Geometry check sheet. Reference: the model listing, model coordinates, mm. A direction names the side the tool comes from. Round coordinates to 2 decimals unless told otherwise and drop trailing zeros. Order: outer loops, then holes, each group sorted by start corner. A loop starts at its lowest first (then second) coordinate and runs counter-clockwise, first axis right, second up.
(1) Sectioned sample at A-A (z = 2.5). Record the boundary of the cut face in (x, y).
(2) Material ranges on line 1 along X through (y, z) = (18.95, 6.25); line 2 along Y through (x, z) = (5, 1.75); line 3 along X through (y, z) = (14.5, 7.5), recorded low to high.
(3) Release check for a two-part mould opening along Y. For faces 4 (the face through (21, 22.3, 11)), 5 (the face through (22.4, 9, 6)), 6 (the face through (11, 11, 0)) record: +Y half, -Y half, draft (parallel to the pull), parting line (faces both ways), or undercut.
(4) Sectioned sample at C-C (y = 3). Record the boundary of the cut face in (x, z), plus the area to 3 significant figures.
(5) Sectioned sample at B-B (x = 19). Record the boundary of the cut face in (y, z).
(6) Go/stop test with flat-tipped pins: pin 1 (2 mm diameter, centred on x = -2.42, z = 6.25, fed in from -Y); pin 2 (4 mm diameter, centred on x = 24.5, z = 8, fed in from +Y); pin 3 (0.9 mm diameter, centred on x = 24.5, z = 7, fed in from -Y). Record where each tip stops, or that it passes through.
(7) Sectioned sample at D-D (x = 5.5). Record the boundary of the cut face in (y, z), plus the area to 3 significant figures.
(8) Set-up check for faces 1 (the face through (21, 22.3, 1)), 2 (the face through (12.35, 25.01, 1.29)), 3 (the face through (24, 5, 4.45)): record each of +Z, -Z, +X, -X, +Y, -Y from which the full face is reachable in a straight line by a thin tool's end or side.
from build123d import *

# Parameters (mm, degrees)
SKETCH_1_W          = 22.4
SKETCH_1_H          = 22.3
EXTRUDE_1_DEPTH     = 12.5
SKETCH_5_R          = 6.25
EXTRUDE_4_DEPTH     = 5.5
SKETCH_6_R          = 2.35
EXTRUDE_5_DEPTH     = 3.7
SKETCH_10_W         = 12.5
SKETCH_10_H         = 2.5
EXTRUDE_8_DEPTH     = 4.7
SKETCH_11_W         = 12.5
SKETCH_11_H         = 2.5
EXTRUDE_9_DEPTH     = 4.7
SKETCH_12_R         = 0.9
CUT_EXTRUDE_2_DEPTH = 4.7
SKETCH_13_W         = 3.6
SKETCH_13_H         = 1.2
EXTRUDE_10_DEPTH    = 3


with BuildPart() as part:
    # 草图1 → 凸台-拉伸1 (new body)
    with BuildSketch(Plane.XY):
        with Locations((11.2, 11.15)):
            Rectangle(SKETCH_1_W, SKETCH_1_H)
    extrude(amount=EXTRUDE_1_DEPTH)

    # 草图5 → 凸台-拉伸4 (add)
    with BuildSketch(Plane(origin=(0, 22.3, 0), x_dir=(1, 0, 0), z_dir=(0, 1, 0))):
        with Locations(Location((16.15, -6.25, 0), (0, 0, 270))):
            Circle(SKETCH_5_R)
    extrude(amount=EXTRUDE_4_DEPTH)

    # 草图6 → 凸台-拉伸5 (add)
    with BuildSketch(Plane(origin=(0, 27.8, 0), x_dir=(1, 0, 0), z_dir=(0, 1, 0))):
        with Locations(Location((16.15, -6.25, 0), (0, 0, 270))):
            Circle(SKETCH_6_R)
    extrude(amount=EXTRUDE_5_DEPTH)

    # 草图10 → 凸台-拉伸8 (add)
    with BuildSketch(Plane(origin=(22.4, 0, 0), x_dir=(0, 0, -1), z_dir=(1, 0, 0))):
        with Locations((-6.25, 19.55)):
            Rectangle(SKETCH_10_W, SKETCH_10_H)
    extrude(amount=EXTRUDE_8_DEPTH)

    # 草图11 → 凸台-拉伸9 (add)
    with BuildSketch(Plane.ZY):
        with Locations((6.25, 19.55)):
            Rectangle(SKETCH_11_W, SKETCH_11_H)
    extrude(amount=EXTRUDE_9_DEPTH)

    # 草图12 → 切除-拉伸2 (cut)
    with BuildSketch(Plane(origin=(0, 20.8, 0), x_dir=(1, 0, 0), z_dir=(0, 1, 0))):
        with Locations(Location((-2.422009123, -6.25, 0), (0, 0, 270))):
            Circle(SKETCH_12_R)
        with Locations(Location((24.822009123, -6.25, 0), (0, 0, 270))):
            Circle(SKETCH_12_R)
    extrude(amount=-CUT_EXTRUDE_2_DEPTH, mode=Mode.SUBTRACT)

    # 草图13 → 凸台-拉伸10 (add)
    with BuildSketch(Plane(origin=(22.4, 0, 0), x_dir=(0, 0, -1), z_dir=(1, 0, 0))):
        with Locations((-6.25, 5.3)):
            Rectangle(SKETCH_13_W, SKETCH_13_H)
    extrude(amount=EXTRUDE_10_DEPTH)


solid = part.part
Answer below:
1. outline: (-4.7, 18.3) - (0, 18.3) - (0, 0) - (22.4, 0) - (22.4, 18.3) - (27.1, 18.3) - (27.1, 20.8) - (22.4, 20.8) - (22.4, 22.3) - (21.15, 22.3) - (21.15, 27.8) - (11.15, 27.8) - (11.15, 22.3) - (0, 22.3) - (0, 20.8) - (-4.7, 20.8) - close
2. line 1: x = -4.7 to -3.32, -1.52 to 23.92, 25.72 to 27.1
2. line 2: y = 0 to 22.3
2. line 3: x = 0 to 22.4
3. face 4: +Y half
3. face 5: undercut
3. face 6: draft
4. outline: (0, 0) - (22.4, 0) - (22.4, 12.5) - (0, 12.5) - close
4. area: 280 mm2
5. outline: (0, 0) - (22.3, 0) - (22.3, 0.69) - (27.8, 0.69) - (27.8, 11.81) - (22.3, 11.81) - (22.3, 12.5) - (0, 12.5) - close
6. pin 1: stops at y = 18.3
6. pin 2: stops at y = 20.8
6. pin 3: stops at y = 4.7
7. outline: (0, 0) - (22.3, 0) - (22.3, 12.5) - (0, 12.5) - close
7. area: 279 mm2
8. face 1: -Z, +X, +Y
8. face 2: +Y
8. face 3: -Z, +X, -Y
